Geometry check sheet. Reference: the model listing, model coordinates, mm. Coordinates: 2 decimals unless noted, no trailing zeros. Write each loop counter-clockwise with the first axis right and the second up, starting at its lowest first coordinate (ties: lowest second). Pieces come first, ordered by that corner, then holes. Notation, with made-up numbers: (-14.5, 59) -> (12.5, 59) arc R13 cw to (12.5, 77) -> close; hole circle Ø9 at (17.5, 34.5). An arc over 180 degrees is marked (long way). One line per question, with ' | ' between items.
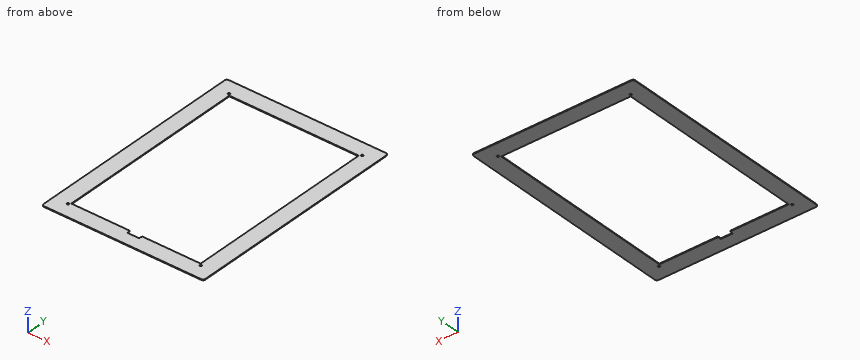
```python
from build123d import *

# Parameters (mm, degrees)
F0_W     = 341.3125
F0_H     = 473.075
F0_R     = 2.15265
F0_W_2   = 273.05
F0_H_2   = 404.8125
F1_DEPTH = 1.5875
F2_R     = 4.7625
F3_W     = 25.4
F3_H     = 7.14375
F4_DEPTH = 1.5875
F5_SIZE  = 1.5875


with BuildPart() as f1:
    # F0 (on Top) → F1 (new body)
    with BuildSketch(Plane.XY):
        Rectangle(F0_W, F0_H)
        with Locations((-140.49375, -206.375)):
            Circle(F0_R, mode=Mode.SUBTRACT)
        with Locations((140.49375, -206.375)):
            Circle(F0_R, mode=Mode.SUBTRACT)
        Rectangle(F0_W_2, F0_H_2, mode=Mode.SUBTRACT)
        with Locations((-140.49375, 206.375)):
            Circle(F0_R, mode=Mode.SUBTRACT)
        with Locations((140.49375, 206.375)):
            Circle(F0_R, mode=Mode.SUBTRACT)
    extrude(amount=F1_DEPTH)

    # F2
    f2_edges = [f1.edges().sort_by_distance(p)[0] for p in [
        (-170.65625, 236.5375, 0.79375),
        (170.65625, 236.5375, 0.79375),
        (170.65625, -236.5375, 0.79375),
        (-170.65625, -236.5375, 0.79375),
    ]]
    fillet(f2_edges, radius=F2_R)

    # F3 (on face) → F4 (cut, through all)
    with BuildSketch(Plane.XY.offset(1.5875)):
        with Locations((0, -205.978125)):
            Rectangle(F3_W, F3_H)
    extrude(amount=-F4_DEPTH, mode=Mode.SUBTRACT)

    # F5
    f5_edges = [f1.edges().sort_by_distance(p)[0] for p in [
        (12.7, -202.40625, 0.79375),
        (-12.7, -202.40625, 0.79375),
    ]]
    chamfer(f5_edges, length=F5_SIZE)


solid = f1.part
```
(1) Cross-section at B-B (y = -159.5). Record the cut outline in (x, z) (1 decimal).
Answers below:
outline: (-170.7, 0) -> (-136.5, 0) -> (-136.5, 1.6) -> (-170.7, 1.6) -> close; (136.5, 0) -> (170.7, 0) -> (170.7, 1.6) -> (136.5, 1.6) -> close
(2) Material ranges on line 1 (Y direction, x = 62, z = 0.2); line 2 (X direction, y = -164.5, z = 1) (3 decimals); line 3 (Y direction, x = -6, z = 1.4), recorded low to high.
Answers below:
line 1: y = -236.54 to -202.41, 202.41 to 236.54 | line 2: x = -170.656 to -136.525, 136.525 to 170.656 | line 3: y = -236.54 to -209.55, 202.41 to 236.54
(3) Cross-section at C-C (z = 1.15). Count the separate pieces of the cut face and the enclosed holes in it, plus the area to 3 significant figures.
Answers below:
separate pieces: 1 | enclosed holes: 5 | area: 50,700 mm²
(4) Cross-section at A-A (x = 96). Record the cut outline in (y, z).
Answers below:
outline: (-236.54, 0) -> (-202.41, 0) -> (-202.41, 1.59) -> (-236.54, 1.59) -> close; (202.41, 0) -> (236.54, 0) -> (236.54, 1.59) -> (202.41, 1.59) -> close
